CAD build for the part. Positions are in the model's coordinates, mm. Round coordinates to 2 decimals unless told otherwise and drop trailing zeros. Order: outer loops, then holes, each group sorted by start corner. A loop starts at its lowest first (then second) coordinate and runs counter-clockwise, first axis right, second up. Notation, with made-up numbers: M -30.5,1 L -9.5,1 A15 cw -9.5,24 Z; hole C 73,-7 d9. An arc over 180 degrees is marked long. Answer as CSV lines item,"result". Start each with the question number.
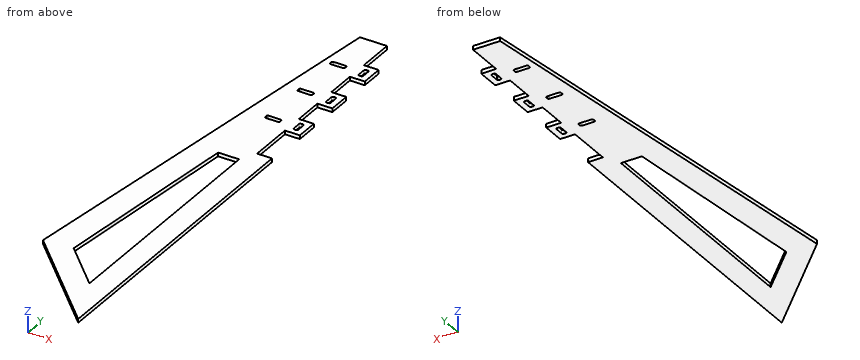
Autodesk Inventor part; units mm, degrees
ref_plane "YZ Plane" through (0, 0, 0) normal (1, 0, 0) x (0, 1, 0)
ref_plane "XZ Plane" through (0, 0, 0) normal (0, 1, 0) x (-1, 0, 0)
ref_plane "XY Plane" through (0, 0, 0) normal (0, 0, 1) x (1, 0, 0)
sketch "Szkic1" plane through (0, 0, 0) normal (0, 0, 1) x (1, 0, 0)
  line L0 (176.3308, 486.6406) -> (176.3308, 940.0878) construction
  line L1 (146.3308, 1046.0878) -> (146.3308, 531.0878) construction
  line L2 (246.3308, 494.0715) -> (246.3308, 1046.1041) construction
  line L3 (-96.6896, 915.5533) -> (106.9406, 915.5533) construction
  line L4 (106.9406, 482.7854) -> (106.9406, 1180.5533)
  line L5 (106.9406, 482.7854) -> (-19.1, 609.3854)
  line L6 (50.6014, 1180.5533) -> (-19.1, 609.3854)
  line L7 (19.8894, 612.8224) -> (76.2561, 1146.5389)
  line L8 (76.2561, 1146.5389) -> (76.2561, 556.2056)
  line L9 (43.2451, 833.9694) -> (8.8194, 838.1705) construction
  line L10 (76.2561, 556.2056) -> (54.9566, 535.0002) construction
  line L11 (76.2561, 613.2072) -> (106.9406, 613.2072) construction
  line L12 (76.2561, 556.2056) -> (19.8894, 612.8224)
  line L13 (14.654, 575.0721) -> (120.72, 469.0061) construction
  line L14 (10.3406, 579.3854) -> (14.654, 575.0721) construction
  line L15 (-19.1, 622) -> (-19.1, 0) construction
  line L16 (-8.2, 622) -> (-16.1, 622) construction
  line L17 (-6.6931, 622) -> (-1.5069, 622) construction
  line L18 (-19.1, 622) -> (-16.1, 622) construction
  line L19 (7.9, 622) -> (0, 622) construction
  line L20 (10.9, 621.8118) -> (36.4266, 596.2853) construction
  line L21 (36.4266, 596.2853) -> (142.1601, 489.8877) construction
  line L22 (48.0033, 879.023) -> (76.2561, 879.023)
  line L23 (91.9406, 1180.5533) -> (424.3104, 1180.5533) construction
  line L24 (106.9406, 915.5533) -> (383.3104, 915.5533) construction
  line L25 (91.9406, 1180.5533) -> (50.6014, 1180.5533)
  line L26 (106.9406, 1180.5533) -> (50.6014, 1180.5533)
  point P0 (0, 0)
  dimension "d0" = 30
  dimension "d1" = 100
ref_plane "Płaszczyzna konstrukcyjna1" through (0, 0, 5) normal (0, 0, 1) x (1, 0, 0)
extrude "Wyciągnięcie proste4" add sketch "Szkic1" along normal blind 5 contours L5 L6 L25 L26 L4 | L7 L8 L22
sketch "Szkic3" plane through (0, 0, 0) normal (0, 0, -1) x (-1, 0, 0)
  line L0 (-48.0033, 879.023) -> (-19.8894, 612.8224)
  line L1 (-19.8894, 612.8224) -> (-76.2561, 556.2056)
  line L2 (-76.2561, 556.2056) -> (-76.2561, 879.023)
  line L3 (-76.2561, 879.023) -> (-48.0033, 879.023)
  line L4 (-106.9406, 1180.5533) -> (-106.9406, 482.7854)
  line L5 (-106.9406, 482.7854) -> (19.1, 609.3854)
  line L6 (19.1, 609.3854) -> (-50.6014, 1180.5533)
  line L7 (-50.6014, 1180.5533) -> (-106.9406, 1180.5533) construction
  line L8 (-106.9406, 482.7854) -> (-106.9406, 1180.5533)
  line L9 (-106.9406, 1060.5533) -> (-86.9406, 1060.5533)
  line L10 (-86.9406, 1060.5533) -> (-86.9406, 1100.5533)
  line L11 (-86.9406, 1100.5533) -> (-106.9406, 1100.5533)
  line L12 (-106.9406, 1100.5533) -> (-106.9406, 1060.5533)
  line L13 (-106.9406, 1130.5533) -> (-86.9406, 1130.5533)
  line L14 (-86.9406, 1130.5533) -> (-86.9406, 1180.5533)
  line L15 (-86.9406, 1180.5533) -> (-106.9406, 1180.5533)
  line L16 (-106.9406, 1180.5533) -> (-106.9406, 1130.5533)
  line L17 (-106.9406, 1030.5533) -> (-86.9406, 1030.5533)
  line L18 (-86.9406, 1030.5533) -> (-86.9406, 990.5533)
  line L19 (-86.9406, 990.5533) -> (-106.9406, 990.5533)
  line L20 (-106.9406, 990.5533) -> (-106.9406, 1030.5533)
  line L21 (-226, 915.5533) -> (53, 915.5533) construction
  line L22 (-86.9406, 990.5533) -> (-106.9406, 990.5533)
  line L23 (-106.9406, 990.5533) -> (-106.9406, 960.5533)
  line L24 (-106.9406, 960.5533) -> (-86.9406, 960.5533)
  line L25 (-86.9406, 960.5533) -> (-106.9406, 960.5533)
  line L26 (-106.9406, 960.5533) -> (-106.9406, 900.5533)
  line L27 (-106.9406, 900.5533) -> (-86.9406, 900.5533)
  line L28 (-86.9406, 900.5533) -> (-86.9406, 960.5533)
  line L29 (-98.9406, 968.0533) -> (-92.9406, 968.0533)
  line L30 (-92.9406, 968.0533) -> (-92.9406, 983.0533)
  line L31 (-92.9406, 983.0533) -> (-98.9406, 983.0533)
  line L32 (-98.9406, 983.0533) -> (-98.9406, 968.0533)
  line L33 (-98.9406, 1038.0533) -> (-92.9406, 1038.0533)
  line L34 (-92.9406, 1038.0533) -> (-92.9406, 1053.0533)
  line L35 (-92.9406, 1053.0533) -> (-98.9406, 1053.0533)
  line L36 (-98.9406, 1053.0533) -> (-98.9406, 1038.0533)
  line L37 (-98.9406, 1108.0533) -> (-92.9406, 1108.0533)
  line L38 (-92.9406, 1108.0533) -> (-92.9406, 1123.0533)
  line L39 (-92.9406, 1123.0533) -> (-98.9406, 1123.0533)
  line L40 (-98.9406, 1123.0533) -> (-98.9406, 1108.0533)
  point P0 (0, 0)
  dimension "d28" = 265
  dimension "d30" = 30
  dimension "d31" = 30
  dimension "d32" = 40
  dimension "d33" = 40
  dimension "d34" = 30
  dimension "d38" = 20
  dimension "d39" = 6
  dimension "d40" = 15
  dimension "d41" = 6
  dimension "d42" = 15
  dimension "d43" = 6
  dimension "d44" = 15
  dimension "d45" = 7.5
  dimension "d46" = 7.5
  dimension "d47" = 7.5
  dimension "d48" = 8
  dimension "d49" = 8
  dimension "d64" = 50
extrude "Wyciągnięcie proste5" cut sketch "Szkic3" against normal blind 5 contours L15 L14 L13 L4 | L24 L28 L27 L4 | L17 L18 L19 L4 | L11 L10 L9 L4 | L32 L31 L30 L29 | L36 L35 L34 L33 | L40 L39 L38 L37
fillet "Zaokrąglenie1" radius 2 12 edges at (98.9406, 968.0533, 2.5) (92.9406, 968.0533, 2.5) (92.9406, 983.0533, 2.5) (98.9406, 983.0533, 2.5) (98.9406, 1053.0533, 2.5) (98.9406, 1038.0533, 2.5) (92.9406, 1038.0533, 2.5) (92.9406, 1053.0533, 2.5) (92.9406, 1123.0533, 2.5) (92.9406, 1108.0533, 2.5) (98.9406, 1108.0533, 2.5) (98.9406, 1123.0533, 2.5)
sketch "Szkic4" plane through (0, 0, 5) normal (0, 0, 1) x (1, 0, 0)
  line L0 (19.8894, 612.8224) -> (48.0033, 879.023)
  line L1 (48.0033, 879.023) -> (76.2561, 879.023)
  line L2 (76.2561, 879.023) -> (76.2561, 556.2056)
  line L3 (76.2561, 556.2056) -> (19.8894, 612.8224)
  line L4 (92.9406, 1110.0533) -> (92.9406, 1121.0533)
  arc A0 (94.9406, 1123.0533) -> (92.9406, 1121.0533) centre (94.9406, 1121.0533) ccw
  line L5 (94.9406, 1123.0533) -> (96.9406, 1123.0533)
  arc A1 (98.9406, 1121.0533) -> (96.9406, 1123.0533) centre (96.9406, 1121.0533) ccw
  line L6 (98.9406, 1121.0533) -> (98.9406, 1110.0533)
  arc A2 (96.9406, 1108.0533) -> (98.9406, 1110.0533) centre (96.9406, 1110.0533) ccw
  line L7 (96.9406, 1108.0533) -> (94.9406, 1108.0533)
  arc A3 (92.9406, 1110.0533) -> (94.9406, 1108.0533) centre (94.9406, 1110.0533) ccw
  line L8 (92.9406, 970.0533) -> (92.9406, 981.0533)
  arc A4 (94.9406, 983.0533) -> (92.9406, 981.0533) centre (94.9406, 981.0533) ccw
  line L9 (94.9406, 983.0533) -> (96.9406, 983.0533)
  arc A5 (98.9406, 981.0533) -> (96.9406, 983.0533) centre (96.9406, 981.0533) ccw
  line L10 (98.9406, 981.0533) -> (98.9406, 970.0533)
  arc A6 (96.9406, 968.0533) -> (98.9406, 970.0533) centre (96.9406, 970.0533) ccw
  line L11 (96.9406, 968.0533) -> (94.9406, 968.0533)
  arc A7 (92.9406, 970.0533) -> (94.9406, 968.0533) centre (94.9406, 970.0533) ccw
  line L12 (92.9406, 1040.0533) -> (92.9406, 1051.0533)
  arc A8 (94.9406, 1053.0533) -> (92.9406, 1051.0533) centre (94.9406, 1051.0533) ccw
  line L13 (94.9406, 1053.0533) -> (96.9406, 1053.0533)
  arc A9 (98.9406, 1051.0533) -> (96.9406, 1053.0533) centre (96.9406, 1051.0533) ccw
  line L14 (98.9406, 1051.0533) -> (98.9406, 1040.0533)
  arc A10 (96.9406, 1038.0533) -> (98.9406, 1040.0533) centre (96.9406, 1040.0533) ccw
  line L15 (96.9406, 1038.0533) -> (94.9406, 1038.0533)
  arc A11 (92.9406, 1040.0533) -> (94.9406, 1038.0533) centre (94.9406, 1040.0533) ccw
  line L16 (106.9406, 990.5533) -> (86.9406, 990.5533)
  line L17 (86.9406, 990.5533) -> (86.9406, 1030.5533)
  line L18 (86.9406, 1030.5533) -> (106.9406, 1030.5533)
  line L19 (106.9406, 1030.5533) -> (106.9406, 1060.5533)
  line L20 (106.9406, 1060.5533) -> (86.9406, 1060.5533)
  line L21 (86.9406, 1060.5533) -> (86.9406, 1100.5533)
  line L22 (86.9406, 1100.5533) -> (106.9406, 1100.5533)
  line L23 (106.9406, 1100.5533) -> (106.9406, 1130.5533)
  line L24 (106.9406, 1130.5533) -> (86.9406, 1130.5533)
  line L25 (86.9406, 1130.5533) -> (86.9406, 1180.5533)
  line L26 (86.9406, 1180.5533) -> (50.6014, 1180.5533)
  line L27 (50.6014, 1180.5533) -> (-19.1, 609.3854)
  line L28 (-19.1, 609.3854) -> (106.9406, 482.7854)
  line L29 (106.9406, 482.7854) -> (106.9406, 900.5533)
  line L30 (106.9406, 900.5533) -> (86.9406, 900.5533)
  line L31 (86.9406, 900.5533) -> (86.9406, 960.5533)
  line L32 (86.9406, 960.5533) -> (106.9406, 960.5533)
  line L33 (106.9406, 960.5533) -> (106.9406, 990.5533)
  line L34 (51.9406, 972.5533) -> (71.9406, 972.5533)
  line L35 (71.9406, 972.5533) -> (71.9406, 978.5533)
  line L36 (71.9406, 978.5533) -> (51.9406, 978.5533)
  line L37 (51.9406, 978.5533) -> (51.9406, 972.5533)
  line L38 (51.9406, 1042.5533) -> (71.9406, 1042.5533)
  line L39 (71.9406, 1042.5533) -> (71.9406, 1048.5533)
  line L40 (71.9406, 1048.5533) -> (51.9406, 1048.5533)
  line L41 (51.9406, 1048.5533) -> (51.9406, 1042.5533)
  line L42 (51.9406, 1112.5533) -> (71.9406, 1112.5533)
  line L43 (71.9406, 1112.5533) -> (71.9406, 1118.5533)
  line L44 (71.9406, 1118.5533) -> (51.9406, 1118.5533)
  line L45 (51.9406, 1118.5533) -> (51.9406, 1112.5533)
  point P0 (0, 0)
  dimension "d51" = 20
  dimension "d52" = 6
  dimension "d53" = 20
  dimension "d54" = 6
  dimension "d55" = 20
  dimension "d56" = 6
  dimension "d57" = 64
  dimension "d58" = 64
  dimension "d59" = 12
  dimension "d60" = 15
extrude "Wyciągnięcie proste6" cut sketch "Szkic4" against normal blind 5 contours L37 L36 L35 L34 | L41 L40 L39 L38 | L45 L44 L43 L42
fillet "Zaokrąglenie2" radius 2 12 edges at (51.9406, 972.5533, 2.5) (71.9406, 972.5533, 2.5) (71.9406, 978.5533, 2.5) (51.9406, 978.5533, 2.5) (51.9406, 1048.5533, 2.5) (51.9406, 1042.5533, 2.5) (71.9406, 1042.5533, 2.5) (71.9406, 1048.5533, 2.5) (71.9406, 1118.5533, 2.5) (51.9406, 1118.5533, 2.5) (71.9406, 1112.5533, 2.5) (51.9406, 1112.5533, 2.5)
equation "\"d30\" = d34"
equation "\"d31\" = d34"
equation "\"d32\" = d33"
equation "\"d39\" = d43"
equation "\"d40\" = d44"
equation "\"d41\" = d43"
equation "\"d42\" = d40"
equation "\"d46\" = d45"
equation "\"d47\" = d46"
equation "\"d49\" = d48"
equation "\"d53\" = d51"
equation "\"d55\" = d51"
equation "\"d58\" = d57"
properties part number "bok"
Q1. Band-saw the part on D-D, the plane y = 1090. Write the cut outline in (x, z), then the cut area to 3 significant figures.
Q2. Drop flat-ended pins along their axis: P1, Ø2.5, axis at x = 96.5, z = 1.5, coming from the +Y side; P2, Ø2, axis at y = 848.5, z = 2.5, coming from the -X side; P3, Ø2, axis at y = 1045.5, z = 3.5, coming from the -X side. Give the stop position or say it passes through.
Q3. Band-saw the part on B-B, the plane x = 29. Write the cut outline in (y, z), then the cut area to 3 significant figures.
Q4. Band-saw the part on C-C, the plane z = 3.15. Count the separate pieces of the cut face and the enclosed holes in it, then the cut area to 3 significant figures.
Q5. Band-saw the part on A-A, the plane y = 669.5. Write the cut outline in (x, z).
Q6. Probe line 1 along X through (y, z) = (1116.5, 2.85); line 2 along Y through (x, z) = (60, 1.45); line 3 along Y through (x, z) = (100.5, 1.65). List the from-to ranges inside material, lowest first. Write a range as from..to.
Answer:
1,outline,"M 39.55,0 L 86.94,0 L 86.94,5 L 39.55,5 Z"
1,area,"237 mm^2"
2,P1,"stops at y = 1130.55"
2,P2,"stops at x = 9.96"
2,P3,"stops at x = 34"
3,outline,"M 561.07,0 L 603.67,0 L 603.67,5 L 561.07,5 Z; M 699.09,0 L 1003.54,0 L 1003.54,5 L 699.09,5 Z"
3,area,"1,740 mm^2"
4,separate pieces,"1"
4,enclosed holes,"7"
4,area,"42,800 mm^2"
5,outline,"M -11.76,0 L 25.88,0 L 25.88,5 L -11.76,5 Z; M 76.26,0 L 106.94,0 L 106.94,5 L 76.26,5 Z"
6,line 1,"x = 42.78..51.94, 71.94..92.94, 98.94..106.94"
6,line 2,"y = 529.93..572.53, 879.02..972.55, 978.55..1042.55, 1048.55..1112.55, 1118.55..1180.55"
6,line 3,"y = 489.25..900.55, 960.55..990.55, 1030.55..1060.55, 1100.55..1130.55"
